```python
from build123d import *

# Parameters (mm, degrees)
SKETCH1_W               = 100
SKETCH1_H               = 60
BOSS_EXTRUDE1_DEPTH     = 6.35
F_3_8_CLEARANCE_HOLE1_D = 10.0838
FILLET1_R               = 10


with BuildPart() as part:
    # Sketch1 → Boss-Extrude1 (new body)
    with BuildSketch(Plane(origin=(0, 0, 0), x_dir=(1, 0, 0), z_dir=(0, 1, 0))):
        Rectangle(SKETCH1_W, SKETCH1_H)
    extrude(amount=BOSS_EXTRUDE1_DEPTH)

    # 3/8 Clearance Hole1 (through all)
    with Locations(Plane(origin=(0, 6.35, 0), x_dir=(1, 0, 0), z_dir=(0, 1, 0))):
        with Locations((0, 15), (0, -15)):
            Hole(F_3_8_CLEARANCE_HOLE1_D / 2)

    # Fillet1
    fillet1_edges = [part.edges().sort_by_distance(p)[0] for p in [
        (-50, 3.175, 30),
        (-50, 3.175, -30),
        (50, 3.175, -30),
        (50, 3.175, 30),
    ]]
    fillet(fillet1_edges, radius=FILLET1_R)


solid = part.part
```
Source: CAD feature listing. Evaluate the final solid. Frame: model axes, mm. Coordinates: 2 decimals unless noted, no trailing zeros. Loops run counter-clockwise (first coordinate to the right, second up) from the corner with the lowest first, then second, coordinate; pieces in that order, holes last. Notation, with made-up numbers: (35.25, 85.25) - (92.25, 85.25) arc R5 cw to (92.25, 89.25) - close; hole circle Ø10 at (34.5, -35). An arc over 180 degrees is marked (long way). Answer as CSV lines item,"result".
1. Section B-B (z = 15). Return loops of the section in (x, y), then the cut area to 3 significant figures.
Established:
outline,"(-50, 0) - (-5.04, 0) - (-5.04, 6.35) - (-50, 6.35) - close; (5.04, 0) - (50, 0) - (50, 6.35) - (5.04, 6.35) - close"
area,"571 mm2"
2. Section C-C (y = 1). Return loops of the section in (x, z), then the cut area to 3 significant figures.
Established:
outline,"(-50, -20) arc R10 ccw to (-40, -30) - (40, -30) arc R10 ccw to (50, -20) - (50, 20) arc R10 ccw to (40, 30) - (-40, 30) arc R10 ccw to (-50, 20) - close; hole circle Ø10.08 at (0, -15); hole circle Ø10.08 at (0, 15)"
area,"5,750 mm2"
3. Section A-A (x = 0). Return loops of the section in (y, z).
Established:
outline,"(0, -30) - (6.35, -30) - (6.35, -20.04) - (0, -20.04) - close; (0, -9.96) - (6.35, -9.96) - (6.35, 9.96) - (0, 9.96) - close; (0, 20.04) - (6.35, 20.04) - (6.35, 30) - (0, 30) - close"
4. Contact query for flat-ended pins moving along their axis: pin 1 (6 mm diameter, centred on x = 0, z = 15, fed in from -Y); pin 2 (2 mm diameter, centred on y = 3.5, z = -21.5, fed in from +X). Output: stop coordinate, or through.
Established:
pin 1,"passes through"
pin 2,"stops at x = 49.99"
5. Section D-D (z = -26). Return loops of the section in (x, y).
Established:
outline,"(-48, 0) - (48, 0) - (48, 6.35) - (-48, 6.35) - close"
6. Mould query, pull axis Z, two halves, no side actions, for faces 1 (the cylindrical face through (46.99, 3.22, 27.15)), 2 (the cylindrical face through (46.99, 3.22, -27.15)), 3 (the flat face through (50, 3, 0)), 4 (the cylindrical face through (0.66, 3.13, -20)). Classes: released by +Z, released by -Z, zero draft, split by the parting line, or undercut.
Established:
face 1,"released by +Z"
face 2,"released by -Z"
face 3,"zero draft"
face 4,"undercut"
7. Ray query, line 1 (Z direction, x = 0, y = 5.25); line 2 (X direction, y = 5, z = 17.5); line 3 (X direction, y = 6.25, z = 14.5). Return the intervals inside material, ascending.
Established:
line 1,"z = -30 to -20.04, -9.96 to 9.96, 20.04 to 30"
line 2,"x = -50 to -4.38, 4.38 to 50"
line 3,"x = -50 to -5.02, 5.02 to 50"
